from build123d import *

# Parameters (mm, degrees)
F0_W     = 550
F0_H     = 690
F0_W_2   = 287
F0_H_2   = 157
F0_H_3   = 304
F1_DEPTH = 2
F2_R     = 26.5
F3_DEPTH = 2.001
F5_D     = 3.3
F7_D     = 22
F10_D    = 5.5


with BuildPart() as f1:
    # F0 (on Top) → F1 (new body)
    with BuildSketch(Plane.XY):
        Rectangle(F0_W, F0_H)
        with Locations((0, -93.5)):
            Rectangle(F0_W_2, F0_H_2, mode=Mode.SUBTRACT)
        with Locations((0, 160)):
            Rectangle(F0_W_2, F0_H_3, mode=Mode.SUBTRACT)
    extrude(amount=F1_DEPTH)

    # F2 (on face) → F3 (cut, through all)
    with BuildSketch(Plane.XY.offset(2)):
        with Locations((185, -268)):
            Circle(F2_R)
    extrude(amount=-F3_DEPTH, mode=Mode.SUBTRACT)

    # F5 (through all)
    with Locations(Plane.XY.offset(2)):
        with Locations((135, -218), (235, -218), (235, -318), (135, -318)):
            Hole(F5_D / 2)

    # F7 (through all)
    with Locations(Plane.XY.offset(2)):
        with Locations((-205, -232), (-145, -232), (0, -262), (70, -232), (-205, -292), (-145, -292)):
            Hole(F7_D / 2)

    # F10 (through all)
    with Locations(Plane.XY.offset(2)):
        with Locations((-260, 330), (0, 330), (260, 330), (255.986392498, 110), (252.8937458992, -110), (260, -330), (0, -330), (-260, -330), (-260, -110), (-260, 110)):
            Hole(F10_D / 2)


solid = f1.part
Part model, mm, in its own coordinate system. Give positions to 0.01 mm unless a question says otherwise; leave off trailing zeros. Write each loop counter-clockwise with the first axis right and the second up, starting at its lowest first coordinate (ties: lowest second). Pieces come first, ordered by that corner, then holes.
1) Cut at D-D on y = 236. Write the cut outline in (x, z).
Resolved:
outline: (-275, 0) - (-143.5, 0) - (-143.5, 2) - (-275, 2) - close; (143.5, 0) - (275, 0) - (275, 2) - (143.5, 2) - close
2) Cut at C-C on x = 48. Write the cut outline in (y, z).
Resolved:
outline: (-345, 0) - (-172, 0) - (-172, 2) - (-345, 2) - close; (-15, 0) - (8, 0) - (8, 2) - (-15, 2) - close; (312, 0) - (345, 0) - (345, 2) - (312, 2) - close
3) Cut at A-A on y = -232. Write the cut outline in (x, z).
Resolved:
outline: (-275, 0) - (-216, 0) - (-216, 2) - (-275, 2) - close; (-194, 0) - (-156, 0) - (-156, 2) - (-194, 2) - close; (-134, 0) - (59, 0) - (59, 2) - (-134, 2) - close; (81, 0) - (275, 0) - (275, 2) - (81, 2) - close
4) Probe L1, parallel to Y at x = 21.5, z = 0.3; L2, parallel to Y at x = -260, z = 1.4; L3, parallel to X at y = 231.5, z = 1.4. List the from-to ranges inside material, lowest first.
Resolved:
L1: y = -345 to -172, -15 to 8, 312 to 345
L2: y = -345 to -332.75, -327.25 to -112.75, -107.25 to 107.25, 112.75 to 327.25, 332.75 to 345
L3: x = -275 to -143.5, 143.5 to 275
5) Cut at B-B on z = 0.6. State how many separate pieces and enclosed holes the cut face has, then the cut area to 3 significant figures.
Resolved:
separate pieces: 1
enclosed holes: 23
area: 242,000 mm2
6) Pin check, flat tip, straight feed: pin 1 (3.5 mm diameter, centred on x = -260, y = 110, fed in from -Z). Stop position of the tip, or through.
Resolved:
pin 1: passes through
7) Two-plate mould, pull along X, no slides. Class faces 1 (the face through (-4, 5, 2)), 2 (the face through (-136.89, -284.57, 0.99)), 3 (the face through (158.526, -266.835, 1.014)): released by +X, released by -X, zero draft, split by the parting line, or undercut.
Resolved:
face 1: zero draft
face 2: undercut
face 3: undercut
